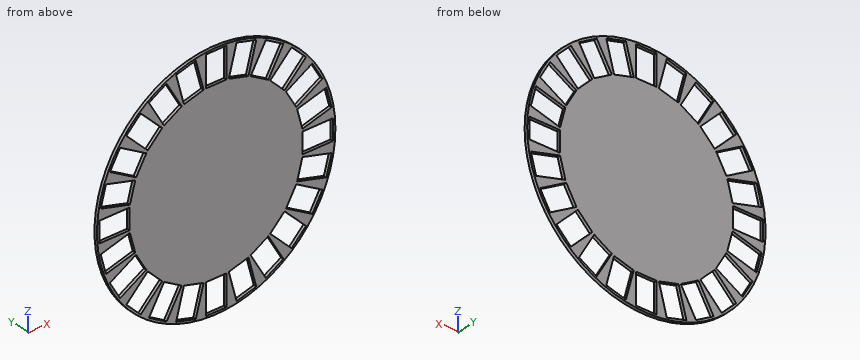
from build123d import *

# Parameters (mm, degrees)
SKETCH1_R           = 120
BOSS_EXTRUDE1_DEPTH = 1.5
SKETCH6_W           = 30.5
SKETCH6_H           = 20.5
SKETCH6_W_2         = 20.5
SKETCH6_H_2         = 30.5
CUT_EXTRUDE1_DEPTH  = 10.5


with BuildPart() as part:
    # Sketch1 → Boss-Extrude1 (new, symmetric)
    with BuildSketch(Plane(origin=(0, 0, 0), x_dir=(1, 0, 0), z_dir=(0, 1, 0))):
        with Locations((98.638798209, 0)):
            Circle(SKETCH1_R)
    extrude(amount=BOSS_EXTRUDE1_DEPTH, both=True)

    # Sketch6 → Cut-Extrude1 (cut)
    with BuildSketch(Plane(origin=(0, 1.5, 0), x_dir=(1, 0, 0), z_dir=(0, 1, 0))):
        with Locations((-3.75, 0)):
            Rectangle(SKETCH6_W, SKETCH6_H)
        Polygon((-12.338659942, 40.347901139), (-17.644450367, 20.5464217), (11.816287335, 12.652440824), (17.122077759, 32.453920263), align=None)
        Polygon((1.885610489, 67.696159493), (-8.364389511, 49.942638716), (18.049385305, 34.692638716), (28.299385305, 52.446159493), align=None)
        Polygon((22.703450772, 90.431036452), (8.207761758, 75.935347437), (29.774518584, 54.368590611), (44.270207598, 68.864279625), align=None)
        Polygon((48.696159493, 107.00318772), (30.942638716, 96.75318772), (46.192638716, 70.339412904), (63.946159493, 80.589412904), align=None)
        Polygon((78.092376509, 116.283248576), (58.29089707, 110.977458152), (66.184877946, 81.51672045), (85.986357385, 86.822510874), align=None)
        with Locations((98.638798209, 102.388798209)):
            Rectangle(SKETCH6_W_2, SKETCH6_H_2)
        Polygon((138.986699348, 110.977458152), (119.185219909, 116.283248576), (111.291239034, 86.822510874), (131.092718473, 81.51672045), align=None)
        Polygon((166.334957703, 96.75318772), (148.581436925, 107.00318772), (133.331436925, 80.589412904), (151.084957703, 70.339412904), align=None)
        Polygon((189.069834661, 75.935347437), (174.574145646, 90.431036452), (153.00738882, 68.864279625), (167.503077834, 54.368590611), align=None)
        Polygon((205.641985929, 49.942638716), (195.391985929, 67.696159493), (168.978211114, 52.446159493), (179.228211114, 34.692638716), align=None)
        Polygon((214.922046785, 20.5464217), (209.616256361, 40.347901139), (180.155518659, 32.453920263), (185.461309084, 12.652440824), align=None)
        with Locations((201.027596418, 0)):
            Rectangle(SKETCH6_W, SKETCH6_H)
        Polygon((209.616256361, -40.347901139), (214.922046785, -20.5464217), (185.461309084, -12.652440824), (180.155518659, -32.453920263), align=None)
        Polygon((195.391985929, -67.696159493), (205.641985929, -49.942638716), (179.228211114, -34.692638716), (168.978211114, -52.446159493), align=None)
        Polygon((174.574145646, -90.431036451), (189.069834661, -75.935347437), (167.503077835, -54.368590611), (153.00738882, -68.864279625), align=None)
        Polygon((148.581436925, -107.00318772), (166.334957703, -96.75318772), (151.084957703, -70.339412904), (133.331436925, -80.589412904), align=None)
        Polygon((119.185219909, -116.283248576), (138.986699348, -110.977458152), (131.092718473, -81.51672045), (111.291239034, -86.822510874), align=None)
        with Locations((98.638798209, -102.388798209)):
            Rectangle(SKETCH6_W_2, SKETCH6_H_2)
        Polygon((58.29089707, -110.977458152), (78.092376509, -116.283248576), (85.986357385, -86.822510874), (66.184877946, -81.51672045), align=None)
        Polygon((30.942638716, -96.75318772), (48.696159493, -107.00318772), (63.946159493, -80.589412904), (46.192638716, -70.339412904), align=None)
        Polygon((8.207761758, -75.935347437), (22.703450772, -90.431036452), (44.270207598, -68.864279625), (29.774518584, -54.368590611), align=None)
        Polygon((-8.364389511, -49.942638716), (1.885610489, -67.696159493), (28.299385305, -52.446159493), (18.049385305, -34.692638716), align=None)
        Polygon((-17.644450367, -20.5464217), (-12.338659942, -40.347901139), (17.122077759, -32.453920263), (11.816287335, -12.652440824), align=None)
    extrude(amount=-CUT_EXTRUDE1_DEPTH, mode=Mode.SUBTRACT)


solid = part.part
Read the model definition and answer for the solid it produces. Units are mm, in the model's axes. Give positions to 0.01 mm unless a question says otherwise; leave off trailing zeros. Loops run counter-clockwise (first coordinate to the right, second up) from the corner with the lowest first, then second, coordinate; pieces in that order, holes last. Notation, with made-up numbers: (-34.75, -9) - (-7.75, -9) arc R16 ccw to (-7.75, 6) - close; hole circle Ø4 at (10.5, 14.5). An arc over 180 degrees is marked (long way). Answer as CSV lines item,"result". Start each with the question number.
1) Each of these flat-tipped pins is pushed along its axis until it touches: pin 1 Ø0.9 at (y, z) = (0, -2.5) entering from -X; pin 2 Ø1.5 at (y, z) = (0, 1) entering from +X; pin 3 Ø0.9 at (x, y) = (97, 0) entering from +Z. Where does it stop, or does it pass through?
2) Straight lines are drawn through the part: L1, parallel to Z at x = 99, y = 0.95; L2, parallel to Z at x = 200.5, y = 0.15; L3, parallel to Z at x = 67, y = 1.25. For each, find the intervals that lie inside material, in ascending order. Write a range as from..to.
3) Find section A-A (x = 161.5). Write down the section's boundary in (y, z), then the cut area to 3 significant figures.
4) Find section B-B (z = 0). Write down the section's boundary in (x, y).
5) Find section C-C (x = -5.5). Write down the section's boundary in (y, z), then the cut area to 3 significant figures.
6) Find section D-D (z = -100). Write down the section's boundary in (x, y), then the cut area to 3 significant figures.
Findings below:
1,pin 1,"x = -21.34"
1,pin 2,"x = 218.64"
1,pin 3,"z = 119.99"
2,L1,"-120..-117.64, -87.14..87.14, 117.64..120"
2,L2,"-63.44..-58.85, -46.97..-37.91, -16.68..-10.25, 10.25..16.68, 37.91..46.97, 58.85..63.44"
2,L3,"-115.75..-113.31, -81.74..81.74, 113.31..115.75"
3,outline,"(-1.5, -102.22) - (1.5, -102.22) - (1.5, -99.54) - (-1.5, -99.54) - close; (-1.5, -88.38) - (1.5, -88.38) - (1.5, -77.36) - (-1.5, -77.36) - close; (-1.5, -60.37) - (1.5, -60.37) - (1.5, 60.37) - (-1.5, 60.37) - close; (-1.5, 77.36) - (1.5, 77.36) - (1.5, 88.38) - (-1.5, 88.38) - close; (-1.5, 99.54) - (1.5, 99.54) - (1.5, 102.22) - (-1.5, 102.22) - close"
3,area,"444 mm^2"
4,outline,"(-21.36, -1.5) - (-19, -1.5) - (-19, 1.5) - (-21.36, 1.5) - close; (11.5, -1.5) - (185.78, -1.5) - (185.78, 1.5) - (11.5, 1.5) - close; (216.28, -1.5) - (218.64, -1.5) - (218.64, 1.5) - (216.28, 1.5) - close"
5,outline,"(-1.5, -59.62) - (1.5, -59.62) - (1.5, -54.9) - (-1.5, -54.9) - close; (-1.5, -48.29) - (1.5, -48.29) - (1.5, -38.52) - (-1.5, -38.52) - close; (-1.5, -17.29) - (1.5, -17.29) - (1.5, -10.25) - (-1.5, -10.25) - close; (-1.5, 10.25) - (1.5, 10.25) - (1.5, 17.29) - (-1.5, 17.29) - close; (-1.5, 38.52) - (1.5, 38.52) - (1.5, 48.29) - (-1.5, 48.29) - close; (-1.5, 54.9) - (1.5, 54.9) - (1.5, 59.62) - (-1.5, 59.62) - close"
5,area,"129 mm^2"
6,outline,"(32.31, -1.5) - (36.57, -1.5) - (36.57, 1.5) - (32.31, 1.5) - close; (52.74, -1.5) - (61.23, -1.5) - (61.23, 1.5) - (52.74, 1.5) - close; (82.46, -1.5) - (88.39, -1.5) - (88.39, 1.5) - (82.46, 1.5) - close; (108.89, -1.5) - (114.82, -1.5) - (114.82, 1.5) - (108.89, 1.5) - close; (136.05, -1.5) - (144.54, -1.5) - (144.54, 1.5) - (136.05, 1.5) - close; (160.71, -1.5) - (164.97, -1.5) - (164.97, 1.5) - (160.71, 1.5) - close"
6,area,"112 mm^2"
